Design review of the part built by this model. Coordinates are the model's own, in mm. A direction names the side the tool comes from. Coordinates: 2 decimals unless noted, no trailing zeros. Answer as a JSON object with one key per item and string values.
from build123d import *

# Parameters (mm, degrees)
F1_DEPTH = 63.5
F2_DEPTH = 25.4
F3_DEPTH = 7.9375


with BuildPart() as f1:
    # F0 (on Front) → F1 (new body, symmetric)
    with BuildSketch(Plane.XZ):
        Polygon((41.275, -9.525), (41.275, 9.525), (22.225, 9.525), (-41.275, 9.525), (-41.275, -9.525), align=None)
    extrude(amount=F1_DEPTH, both=True)

    # F0 (on Front) → F2 (join, symmetric)
    with BuildSketch(Plane.XZ):
        with BuildLine():
            Line((22.225, 9.525), (41.275, 9.525))
            Line((41.275, 9.525), (41.275, 27.0002))
            ThreePointArc((41.275, 27.0002), (45.92468, 38.22552), (57.15, 42.8752))
            Line((57.15, 42.8752), (60.325, 42.8752))
            Line((60.325, 42.8752), (60.325, 61.9252))
            Line((60.325, 61.9252), (57.15, 61.9252))
            add(Edge.make_bspline(
                [(55.649062, 61.892933), (56.146045, 61.905154), (56.646347, 61.915914), (57.15, 61.9252)],
                knots=[110.675556, 110.675556, 110.675556, 110.675556, 111.504536, 111.504536, 111.504536, 111.504536], degree=3))
            ThreePointArc((55.649062, 61.892933), (31.929216, 51.159415), (22.225, 27.0002))
            Line((22.225, 27.0002), (22.225, 9.525))
        make_face()
        Polygon((60.325, 61.9252), (60.325, 42.8752), (85.725, 42.8752), (85.725, 52.3875), (85.725, 61.9252), align=None)
    extrude(amount=F2_DEPTH, both=True)

    # F0 (on Front) → F3 (join, symmetric)
    with BuildSketch(Plane.XZ):
        with BuildLine():
            Line((-41.275, 9.525), (22.225, 9.525))
            Line((22.225, 9.525), (22.225, 27.0002))
            ThreePointArc((22.225, 27.0002), (31.929216, 51.159415), (55.649062, 61.892933))
            add(Edge.make_bspline(
                [(-41.275, 9.525), (-17.894272, 32.578413), (-10.702219, 60.261258), (55.649062, 61.892933)],
                knots=[0, 0, 0, 0, 110.675556, 110.675556, 110.675556, 110.675556], degree=3))
        make_face()
    extrude(amount=F3_DEPTH, both=True)

    # F0 (on Front) → F4 (revolve)
    with BuildSketch(Plane.XZ):
        Polygon((85.725, 52.3875), (85.725, 42.8752), (85.725, 38.1), (111.125, 38.1), (111.125, 66.675), (85.725, 66.675), (85.725, 61.9252), align=None)
    revolve(axis=Axis((85.725, 0, 52.3875), (0, 0, -1)))


solid = f1.part
1) Mouldability with a two-part tool opening along X and no side actions: class faces 1 (the cylindrical face through (45.8, -0.4, 38.1)), 2 (the flat face through (22.225, -17, 18)), 3 (the flat face through (1, 35, 9.525)) as released by +X, released by -X, zero draft, split by the parting line, or undercut.
Taken from the geometry:
{"face 1": "undercut", "face 2": "released by -X", "face 3": "zero draft"}
2) To check wall thickness, follow L1, parallel to Z at x = 90, y = 16 (3 decimals); L2, parallel to X at y = -29.5, z = 6.5 (3 decimals); L3, parallel to Z at x = 28, y = 46.5 (3 decimals). State the ranges of each line that lie inside material, in increasing order.
Taken from the geometry:
{"L1": "z = 38.1 to 66.675", "L2": "x = -41.275 to 41.275", "L3": "z = -9.525 to 9.525"}
3) Tool access review of faces 4 (the flat face through (86, 0, 38.1)), 5 (the flat face through (46, -25.4, 42)), 6 (the flat face through (46, 25.4, 42)), 7 (the flat face through (60, -2, 61.925)), 8 (the flat face through (7, 7.938, 30)): name each direction out of +Z, -Z, +X, -X, +Y, -Y from which nothing blocks a thin tool from reaching the whole face with its end or side.
Taken from the geometry:
{"face 4": "-Z, +X, +Y, -Y", "face 5": "+Z, +X, -X, -Y", "face 6": "+Z, +X, -X, +Y", "face 7": "+Z, -X", "face 8": "+Z, -X, +Y"}
4) Insertion check: pin 1 Ø8 at (x, y) = (6, -14) entering from +Z (3 decimals); pin 2 Ø5 at (y, z) = (-14, 17) entering from -X (3 decimals); pin 3 Ø15 at (x, y) = (97.5, -8.5) entering from -Z. Each pin has a flat end and moves straight along its axis. Give the tip position at first contact, or say it passes through.
Taken from the geometry:
{"pin 1": "stops at z = 9.525", "pin 2": "stops at x = 22.225", "pin 3": "stops at z = 38.1"}
